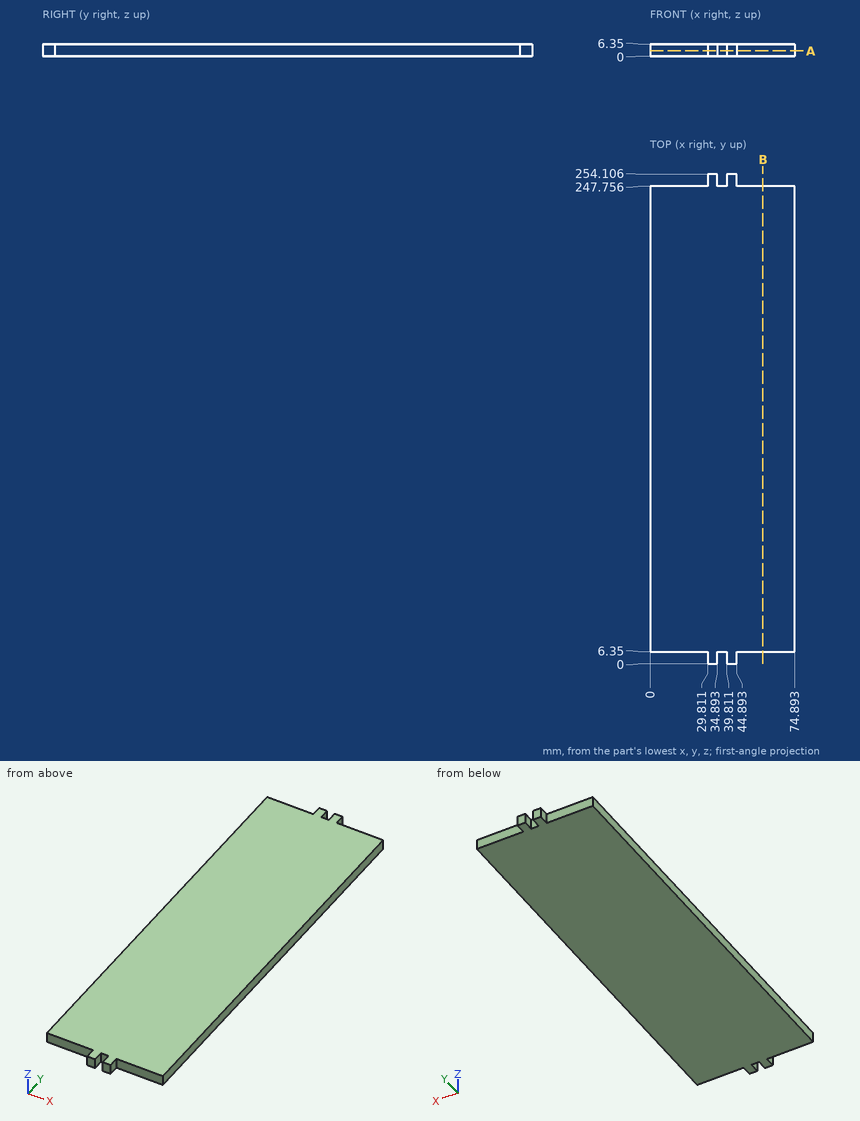
Can you work these out from the drawing? Everything is in mm from the part's minimum corner. Give positions to 0.01 mm unless a question says otherwise; leave off trailing zeros. Order: outer loops, then holes, each group sorted by start corner. A loop starts at its lowest first (then second) coordinate and runs counter-clockwise, first axis right, second up. Notation, with made-up numbers: M 84.25,88 L 122.25,88 A23 ccw 122.25,100 Z; hole C -38,48 d2. An arc over 180 degrees is marked long. Use a Markdown table: item, result. Add a question column.
Item 1: Suppose I cut it at A-A (z = 2.75). List the corners of the cut face in (x, y) for me.
Item 2: Will these pins go through, and if not, where does the flat tip stop? pin 1 (3 mm diameter, centred on x = 8, y = 141, fed in from -Z); pin 2 (1.9 mm diameter, centred on x = 20.5, z = 2, fed in from -Y); pin 3 (1.9 mm diameter, centred on y = 251, z = 2, fed in from +X); pin 4 (3 mm diameter, centred on x = 66.5, z = 4, fed in from +Y).
Item 3: Suppose I cut it at B-B (x = 58.5). List the corners of the cut face in (y, z) for me.
Item 4: If I drill on L1, parallel to Y at x = 26, z = 5.25, over which ranges is the centre line in solid material (lowest first)? Write a range as [from, to].
Answer sheet:
| question | item | result |
|---|---|---|
| 1 | outline | M 0,6.35 L 29.81,6.35 L 29.81,0 L 34.89,0 L 34.89,6.35 L 39.81,6.35 L 39.81,0 L 44.89,0 L 44.89,6.35 L 74.89,6.35 L 74.89,247.76 L 44.89,247.76 L 44.89,254.11 L 39.81,254.11 L 39.81,247.76 L 34.89,247.76 L 34.89,254.11 L 29.81,254.11 L 29.81,247.76 L 0,247.76 Z |
| 2 | pin 1 | stops at z = 0 |
| 2 | pin 2 | stops at y = 6.35 |
| 2 | pin 3 | stops at x = 44.89 |
| 2 | pin 4 | stops at y = 247.76 |
| 3 | outline | M 6.35,0 L 247.76,0 L 247.76,6.35 L 6.35,6.35 Z |
| 4 | L1 | y = [6.35, 247.76] |
